Check sheet for the modelled part. Datum: model origin and axes. Units: mm. Face numbers are marked on the shaded views. A direction names the side the tool comes from. Coordinates: 2 decimals unless noted, no trailing zeros. Loops run counter-clockwise (first coordinate to the right, second up) from the corner with the lowest first, then second, coordinate; pieces in that order, holes last.
```python
from build123d import *

# Parameters (mm, degrees)
F0_W     = 70
F0_H     = 40
F0_R     = 2.25
F0_R_2   = 1.65
F1_DEPTH = 10
F2_R     = 2.25
F2_R_2   = 4.5
F3_DEPTH = 5
F4_R     = 3.75
F5_DEPTH = 5
F6_R     = 1.75
F7_DEPTH = 25
F8_R     = 3.5
F9_DEPTH = 5


with BuildPart() as f1:
    # F0 (on Front) → F1 (new body)
    with BuildSketch(Plane.XZ):
        with Locations((-35, 0)):
            Rectangle(F0_W, F0_H)
        with Locations((-50, -15)):
            Circle(F0_R, mode=Mode.SUBTRACT)
        with Locations((-20, -15)):
            Circle(F0_R, mode=Mode.SUBTRACT)
        with Locations((-39.5, 7)):
            Circle(F0_R_2, mode=Mode.SUBTRACT)
        with Locations((-50, 15)):
            Circle(F0_R, mode=Mode.SUBTRACT)
        with Locations((-30.5, 7)):
            Circle(F0_R_2, mode=Mode.SUBTRACT)
        with Locations((-35, 15)):
            Circle(F0_R_2, mode=Mode.SUBTRACT)
        with Locations((-20, 15)):
            Circle(F0_R, mode=Mode.SUBTRACT)
    extrude(amount=F1_DEPTH)

    # F2 (on face) → F3 (cut)
    with BuildSketch(Plane.XZ.offset(10)):
        with Locations((-50, 15)):
            Circle(F2_R)
        with Locations((-20, 15)):
            Circle(F2_R)
        with Locations((-20, -15)):
            Circle(F2_R)
        with Locations((-50, -15)):
            Circle(F2_R)
        with Locations((-20, 15)):
            Circle(F2_R_2)
        with Locations((-20, 15)):
            Circle(F2_R, mode=Mode.SUBTRACT)
        with Locations((-20, -15)):
            Circle(F2_R_2)
        with Locations((-20, -15)):
            Circle(F2_R, mode=Mode.SUBTRACT)
        with Locations((-50, -15)):
            Circle(F2_R_2)
        with Locations((-50, -15)):
            Circle(F2_R, mode=Mode.SUBTRACT)
        with Locations((-50, 15)):
            Circle(F2_R_2)
        with Locations((-50, 15)):
            Circle(F2_R, mode=Mode.SUBTRACT)
    extrude(amount=-F3_DEPTH, mode=Mode.SUBTRACT)

    # F4 (on face) → F5 (cut)
    with BuildSketch(Plane(origin=(0, 0, 0), x_dir=(-1, 0, 0), z_dir=(0, 1, 0))):
        with Locations((35, 15)):
            Circle(F4_R)
        with Locations((30.5, 7)):
            Circle(F4_R)
        with Locations((39.5, 7)):
            Circle(F4_R)
    extrude(amount=-F5_DEPTH, mode=Mode.SUBTRACT)

    # F6 (on face) → F7 (cut)
    with BuildSketch(Plane.XZ.offset(10)):
        with Locations((-65, 0)):
            Circle(F6_R)
        with Locations((-5, 0)):
            Circle(F6_R)
    extrude(amount=-F7_DEPTH, mode=Mode.SUBTRACT)

    # F8 (on face) → F9 (cut)
    with BuildSketch(Plane(origin=(0, 0, 0), x_dir=(-1, 0, 0), z_dir=(0, 1, 0))):
        with Locations((5, 0)):
            Circle(F8_R)
        with Locations((65, 0)):
            Circle(F8_R)
    extrude(amount=-F9_DEPTH, mode=Mode.SUBTRACT)


solid = f1.part
```
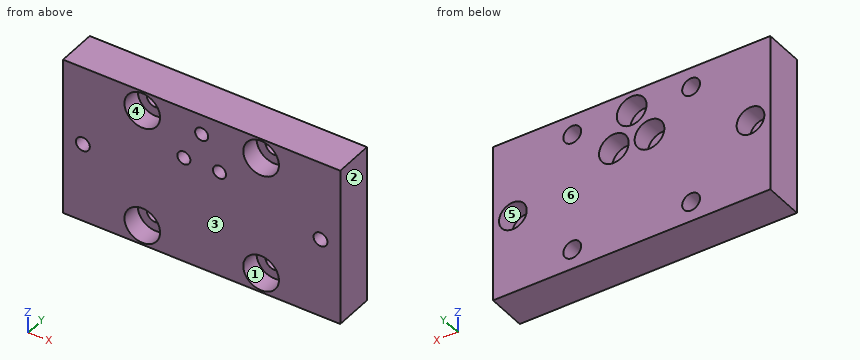
1) Set-up check for the marked faces 4, 5 and 6: record each of +Z, -Z, +X, -X, +Y, -Y from which the full face is reachable in a straight line by a thin tool's end or side.
Answer sheet:
face 4: -Y
face 5: +Y
face 6: +Z, -Z, +X, -X, +Y
2) Mould release check, pull along X, two halves, no side actions. Record for the marked faces 1, 2 and 3: +X half, -X half, draft (parallel to the pull), parting line (faces both ways), or undercut.
Answer sheet:
face 1: undercut
face 2: +X half
face 3: draft
3) Scan lines: line 1 (Z direction, x = -50, y = -2.8); line 2 (Z direction, x = -20, y = -6.75); line 3 (X direction, y = -8.4, z = 7). Record each from-to range of solid material in increasing order.
Answer sheet:
line 1: z = -20 to -17.25, -12.75 to 12.75, 17.25 to 20
line 2: z = -20 to -19.5, -10.5 to 10.5, 19.5 to 20
line 3: x = -70 to -41.15, -37.85 to -32.15, -28.85 to 0
4) Depth check by flat-ended pin: pin 1 (5.5 mm diameter, centred on x = -5, z = 0, fed in from +Y); pin 2 (5 mm diameter, centred on x = -50, z = -15, fed in from -Y). Enter the tip coordinate at first touch or a pass-through.
Answer sheet:
pin 1: stops at y = -5
pin 2: stops at y = -5
5) Section check A-A on x = -5. Enter the section's corners in (y, z), plus the area to 4 significant figures.
Answer sheet:
outline: (-10, -20) - (0, -20) - (0, -3.5) - (-5, -3.5) - (-5, -1.75) - (-10, -1.75) - close; (-10, 1.75) - (-5, 1.75) - (-5, 3.5) - (0, 3.5) - (0, 20) - (-10, 20) - close
area: 347.5 mm2
6) Section check D-D on x = -20. Enter the section's corners in (y, z), plus the area to 3 significant figures.
Answer sheet:
outline: (-10, -20) - (0, -20) - (0, -17.25) - (-5, -17.25) - (-5, -19.5) - (-10, -19.5) - close; (-10, -10.5) - (-5, -10.5) - (-5, -12.75) - (0, -12.75) - (0, 12.75) - (-5, 12.75) - (-5, 10.5) - (-10, 10.5) - close; (-10, 19.5) - (-5, 19.5) - (-5, 17.25) - (0, 17.25) - (0, 20) - (-10, 20) - close
area: 265 mm2
7) Section check B-B on z = 0. Enter the section's corners in (x, y).
Answer sheet:
outline: (-70, -10) - (-66.75, -10) - (-66.75, -5) - (-68.5, -5) - (-68.5, 0) - (-70, 0) - close; (-63.25, -10) - (-6.75, -10) - (-6.75, -5) - (-8.5, -5) - (-8.5, 0) - (-61.5, 0) - (-61.5, -5) - (-63.25, -5) - close; (-3.25, -10) - (0, -10) - (0, 0) - (-1.5, 0) - (-1.5, -5) - (-3.25, -5) - close
8) Section check C-C on y = -2.25. Give the number of separate pieces and of enclosed holes in the cut face, plus the area to 3 significant figures.
Answer sheet:
separate pieces: 1
enclosed holes: 9
area: 2,530 mm2
